from build123d import *

# Parameters (mm, degrees)
F1_ANGLE_BACK = 180.5
F1_ANGLE      = 180.5
F2_R          = 3.5
F3_DEPTH      = 53.34
F3_DEPTH_BACK = 2.54
F6_DEPTH      = 35.56


# Not quite as in the source:
# - a feature names something its author has since deleted; it is built from what else it names


with BuildPart() as f1:
    # F0 (on Front) → F1 (revolve)
    with BuildSketch(Plane.XZ, mode=Mode.PRIVATE) as f1_sk:
        with BuildLine():
            Line((21.5, 36), (21.5, 0))
            Line((21.5, 0), (40.55, 0))
            Line((40.55, 0), (40.55, 2.54))
            Line((40.55, 2.54), (46.9, 2.54))
            Line((46.9, 2.54), (46.9, 32.825))
            ThreePointArc((46.9, 32.825), (45.9700640303, 35.0700640303), (43.725, 36))
            Line((43.725, 36), (21.5, 36))
        make_face()
    revolve(f1_sk.sketch.rotate(Axis((0, 0, -0.0018208164), (0, 0, -1)), -F1_ANGLE_BACK), axis=Axis((0, 0, -0.0018208164), (0, 0, -1)), revolution_arc=F1_ANGLE)

    # F2 (on Front) → F3 (cut, two sides)
    with BuildSketch(Plane.XZ) as f3_sk:
        with Locations((30, 26.5004)):
            Circle(F2_R)
        with Locations((-30, 26.5004)):
            Circle(F2_R)
    extrude(amount=-F3_DEPTH, mode=Mode.SUBTRACT)
    extrude(f3_sk.sketch, amount=F3_DEPTH_BACK, mode=Mode.SUBTRACT)

    # F5 (on offset) → F6 (cut)
    with BuildSketch(Plane.XZ.offset(-50.8)):
        Polygon((36.6991664547, 26.5004), (33.3482832273, 32.3043), (26.6465167727, 32.3043), (23.2956335453, 26.5004), (26.6465167727, 20.6965), (33.3482832273, 20.6965), align=None)
        Polygon((-33.3482832273, 32.3043), (-36.6991664547, 26.5004), (-33.3482832273, 20.6965), (-26.6465167727, 20.6965), (-23.2956335453, 26.5004), (-26.6465167727, 32.3043), align=None)
    extrude(amount=F6_DEPTH, mode=Mode.SUBTRACT)


solid = f1.part
The listing builds one solid part. Answer for the finished solid, in the listing's coordinates (mm). A direction names the side the tool comes from. Coordinates: 2 decimals unless noted, no trailing zeros. Write each loop counter-clockwise with the first axis right and the second up, starting at its lowest first coordinate (ties: lowest second). Pieces come first, ordered by that corner, then holes. Notation, with made-up numbers: (80.5, 1.5) - (93.5, 1.5) arc R17 ccw to (93.5, 18.5) - close; hole circle Ø9 at (-18, 15). An arc over 180 degrees is marked (long way). Put each result on its own line as item: value.
1. A tool of negligible diameter and unlimited length cuts with its end or side. For faces 5 (the face through (-1, 25, 0)), 6 (the face through (-24.948, 28.151, 29.362)), from which of +Z, -Z, +X, -X, +Y, -Y can it reach the whole face along a straight path? Write none if from no direction.
Answer sheet:
face 5: -Z, +X, -X, +Y, -Y
face 6: +Y
2. Find the intervals of material crossed by line 1 along Z through (x, y) = (-30, 12); line 2 along Z through (x, y) = (29, 19.5); line 3 along X through (y, z) = (8, 29.5), in increasing order. Write a range as from..to.
Answer sheet:
line 1: z = 0..23, 30..36
line 2: z = 0..20.7, 32.3..36
line 3: x = -46.21..-31.8, -28.2..-19.96, 19.96..28.2, 31.8..46.21
3. The part is cut by section C-C on y = 9.5. State how many separate pieces and enclosed holes the cut face has, plus the area to 3 significant figures.
Answer sheet:
separate pieces: 2
enclosed holes: 2
area: 1,800 mm^2
4. The part is cut by section B-B on x = 0. Give the vertices of the cut face in (y, z) (3 decimals).
Answer sheet:
outline: (21.5, 0) - (40.55, 0) - (40.55, 2.54) - (46.9, 2.54) - (46.9, 32.825) arc R3.175 ccw to (43.725, 36) - (21.5, 36) - close
5. Flat-ended cylindrical pins translate along their axes: pin 1 Ø3.5 at (x, z) = (31, 29) entering from +Y; pin 2 Ø20.5 at (x, z) = (35, 13) entering from -Y; pin 3 Ø4 at (x, z) = (2.5, 26) entering from -Y. Find the tip coordinate at first contact, or state that the pin passes through.
Answer sheet:
pin 1: stops at y = 15.24
pin 2: stops at y = 0
pin 3: stops at y = 21.02
6. Determine the mould class of faces 1 (the face through (0, 22, 36)), 2 (the face through (30, 24, 32.304)), 3 (the face through (-1.071, 40.536, 1.288)), 4 (the face through (-24.995, 28.151, 23.558)) for opening direction X: pulls with the +X half, pulls with the -X half, needs draft (parallel to the pull), parting line crosses it, or undercut.
Answer sheet:
face 1: needs draft
face 2: undercut
face 3: parting line crosses it
face 4: undercut
7. The part is cut by section A-A on z = 25.5. Give the vertices of the cut face in (x, y).
Answer sheet:
outline: (-46.9, -0.41) - (-33.35, -0.29) - (-33.35, 15.24) - (-36.12, 15.24) - (-36.12, 29.91) arc R46.9 ccw to start; (-26.65, -0.23) - (-21.5, -0.19) arc R21.5 cw (long way) to (21.5, 0) - (26.65, 0) - (26.65, 15.24) - (23.87, 15.24) - (23.87, 40.37) arc R46.9 ccw to (-23.87, 40.37) - (-23.87, 15.24) - (-26.65, 15.24) - close; (33.35, 0) - (46.9, 0) arc R46.9 ccw to (36.12, 29.91) - (36.12, 15.24) - (33.35, 15.24) - close
